from build123d import *

# Parameters (mm, degrees)
SKETCH1_R                   = 12.7
SKETCH1_R_2                 = 4
BOSS_EXTRUDE1_DEPTH         = 3.8
SKETCH2_R                   = 6.34
SKETCH2_R_2                 = 4
BOSS_EXTRUDE2_DEPTH         = 15.2
TAP_DRILL_FOR_M3_TAP1_D     = 2.5
TAP_DRILL_FOR_M3_TAP1_DEPTH = 3.8


with BuildPart() as part:
    # Sketch1 → Boss-Extrude1 (new body)
    with BuildSketch(Plane(origin=(0, 0, 0), x_dir=(1, 0, 0), z_dir=(0, 1, 0))):
        Circle(SKETCH1_R)
        Circle(SKETCH1_R_2, mode=Mode.SUBTRACT)
    extrude(amount=BOSS_EXTRUDE1_DEPTH)

    # Sketch2 → Boss-Extrude2 (add)
    with BuildSketch(Plane(origin=(0, 3.8, 0), x_dir=(1, 0, 0), z_dir=(0, 1, 0))):
        Circle(SKETCH2_R)
        Circle(SKETCH2_R_2, mode=Mode.SUBTRACT)
    extrude(amount=BOSS_EXTRUDE2_DEPTH)

    # Tap Drill for M3 Tap1
    with Locations(Plane(origin=(-8.25, 0, 4.763139721), x_dir=(0, 0, -1), z_dir=(0, -1, 0))):
        with Locations((0, 0), (0, 16.5), (14.289419163, 8.25)):
            Hole(TAP_DRILL_FOR_M3_TAP1_D / 2, depth=TAP_DRILL_FOR_M3_TAP1_DEPTH)


solid = part.part
Check sheet for the modelled part. Datum: model origin and axes. Units: mm. A direction names the side the tool comes from. Give positions to 0.01 mm unless a question says otherwise; leave off trailing zeros. Write each loop counter-clockwise with the first axis right and the second up, starting at its lowest first coordinate (ties: lowest second). Pieces come first, ordered by that corner, then holes. Notation, with made-up numbers: M -2,46.5 L 41,46.5 A20 ccw 41,62.5 Z; hole C -5,-11.75 d1. An arc over 180 degrees is marked long. Use one line per item in the form item = value.
(1) Section check A-A on x = 0. Record the boundary of the cut face in (y, z).
Answer block:
outline = M 0,-12.7 L 3.8,-12.7 L 3.8,-10.78 L 0,-10.78 Z; M 0,-8.28 L 3.8,-8.28 L 3.8,-6.34 L 19,-6.34 L 19,-4 L 0,-4 Z; M 0,4 L 19,4 L 19,6.34 L 3.8,6.34 L 3.8,12.7 L 0,12.7 Z
(2) Material ranges on line 1 along Z through (x, y) = (0, 10); line 2 along Y through (x, z) = (3.25, 11.75), recorded low to high.
Answer block:
line_1 = -6.34 to -4, 4 to 6.34
line_2 = 0 to 3.8
(3) Section check B-B on z = 0. Record the boundary of the cut face in (x, y), plus the area to 3 significant figures.
Answer block:
outline = M -12.7,0 L -4,0 L -4,19 L -6.34,19 L -6.34,3.8 L -12.7,3.8 Z; M 4,0 L 12.7,0 L 12.7,3.8 L 6.34,3.8 L 6.34,19 L 4,19 Z
area = 137 mm2
(4) Depth check by flat-ended pin: P1, Ø5, axis at x = -4.5, y = 8.5, coming from the -Z side; P2, Ø4, axis at y = 7, z = 2.5, coming from the -X side; P3, Ø2, axis at x = -0.5, y = 10, coming from the -Z side. Enter the tip coordinate at first touch or a pass-through.
Answer block:
P1 = -6.02
P2 = -6.32
P3 = -6.34
(5) Section check D-D on y = 1.75. Record the boundary of the cut face in (x, z).
Answer block:
outline = C 0,0 d25.4; hole C -8.25,4.76 d2.5; hole C 0,0 d8; hole C 0,-9.53 d2.5; hole C 8.25,4.76 d2.5
(6) Draft check along X on faces 1 (the cylindrical face through (-2.75, 1.87, 12.4)), 2 (the cylindrical face through (-9.47, 1.93, 4.49)), 3 (the flat face through (1.3, 19, 4.1)). Enter one of: pulls with the +X half, pulls with the -X half, needs draft (parallel to the pull), parting line crosses it, or undercut.
Answer block:
face_1 = parting line crosses it
face_2 = undercut
face_3 = needs draft
(7) Section check C-C on x = -9. Record the boundary of the cut face in (y, z), plus the area to 3 significant figures.
Answer block:
outline = M 0,-8.96 L 3.8,-8.96 L 3.8,3.76 L 0,3.76 Z; M 0,5.76 L 3.8,5.76 L 3.8,8.96 L 0,8.96 Z
area = 60.5 mm2
(8) Tool access check on faces 4 (the cylindrical face through (0.055, 1.927, -10.775)), 5 (the cylindrical face through (-5, 11.3, 3.9)). Record the directions out of +Z, -Z, +X, -X, +Y, -Y that give a thin tool (end or side, any length) a straight path to the whole face; none if there is none.
Answer block:
face_4 = +Y, -Y
face_5 = +Y
